Could you check a few things on this model? Use its own coordinates, in mm. A direction names the side the tool comes from. Give positions to 0.01 mm unless a question says otherwise; leave off trailing zeros. Write each loop counter-clockwise with the first axis right and the second up, starting at its lowest first coordinate (ties: lowest second). Pieces come first, ordered by that corner, then holes. Notation, with made-up numbers: M 4,70 L 17,70 A26 cw 17,99 Z; hole C 75.25,86 d11. An arc over 180 degrees is marked long. Answer as CSV lines item,"result". Start each with the question number.
from build123d import *

# Parameters (mm, degrees)
FILLET1_R           = 11
FILLET2_R           = 1
BOSS_EXTRUDE1_DEPTH = 10.425
CHAMFER1_SIZE       = 0.35


with BuildPart() as part:
    # Sketch1 → Revolve1 (revolve)
    with BuildSketch(Plane.XY, mode=Mode.PRIVATE) as revolve1_sk:
        with BuildLine():
            Line((0, 0), (8.5, 0))
            Line((8.5, 0), (8.5, 1))
            Line((8.5, 1), (5, 8))
            Line((5, 8), (4, 23))
            Line((4, 23), (3.5, 24))
            Line((3.5, 24), (2.5, 24))
            add(Edge.make_bspline(
                [(2.5, 24), (1.3, 23.5), (0, 23.5)],
                knots=[0, 0, 0, 1, 1, 1], degree=2))
            Line((0, 23.5), (0, 0))
        make_face()
    revolve(revolve1_sk.sketch.rotate(Axis((0, 23.5, 0), (0, -1, 0)), 180), axis=Axis((0, 23.5, 0), (0, -1, 0)))

    # Fillet1
    fillet1_edges = [part.edges().sort_by_distance(p)[0] for p in [
        (5, 8, 0),
    ]]
    fillet(fillet1_edges, radius=FILLET1_R)

    # Fillet2
    fillet2_edges = [part.edges().sort_by_distance(p)[0] for p in [
        (2.5, 24, 0),
        (3.5, 24, 0),
        (4, 23, 0),
        (8.5, 1, 0),
    ]]
    fillet(fillet2_edges, radius=FILLET2_R)

    # Sketch3 → Cut-Revolve1 (revolve, cut)
    with BuildSketch(Plane.XY):
        Polygon((0, 0), (3.875, 0), (3.875, 6.5), (3.05, 7.325), (3.05, 17.75), (0, 17.75), align=None)
    revolve(axis=Axis((0, 17.75, 0), (0, -1, 0)), mode=Mode.SUBTRACT)

    # Sketch4 → Boss-Extrude1 (add)
    with BuildSketch(Plane.XZ.offset(-17.75)):
        with BuildLine():
            Line((-2.655654345, 1.5), (2.655654345, 1.5))
            ThreePointArc((2.655654345, 1.5), (0, 3.05), (-2.655654345, 1.5))
        make_face()
        with BuildLine():
            ThreePointArc((-0.099986562, -3.048360656), (0, -3.05), (0.099986562, -3.048360656))
            ThreePointArc((0.099986562, -3.048360656), (0, -2.95), (-0.099986562, -3.048360656))
        make_face()
    extrude(amount=BOSS_EXTRUDE1_DEPTH)

    # Chamfer1
    # the kernel refuses this chamfer: 0.35 mm, written as the material it takes off along each edge
    with BuildSketch(Plane(origin=(-3.555743391, 7.325, 1.5), x_dir=(0, 0.9996219169112968, -0.027495876610586154), z_dir=(1, 0, 0))) as chamfer1_piece_1_section:
        Polygon((CHAMFER1_SIZE * 0.999621916911, CHAMFER1_SIZE * 0.0274958766106), (-CHAMFER1_SIZE * 0.0274958766106, CHAMFER1_SIZE * 0.999621916911), (0, 0), align=None)
    chamfer1_piece_1 = extrude(amount=7.111486782, mode=Mode.PRIVATE)
    chamfer1_piece_1 = chamfer1_piece_1 & Plane(origin=(0, 7.499624527, 0), x_dir=(1, 0, 0), z_dir=(0, 1, 0)) * Cylinder(3.05, 16, mode=Mode.PRIVATE)
    add(chamfer1_piece_1, mode=Mode.SUBTRACT)


solid = part.part
1. Thinking about a two-plate mould opening in Y: for faces 3 (the conical face through (-5.825, 5.787, -1.834)), 4 (the flat face through (4, 0, 2)), 5 (the cylindrical face through (-0.504, 3.296, 3.842)), which applies, pulls with the +Y half, pulls with the -Y half, needs draft (parallel to the pull), parting line crosses it, or undercut?
2. Imagine slicing it at A-A, the plane y = 12.5. Please give me the cut outline in (x, z), plus the area to 3 significant figures.
3. Will these pins go through, and if not, where does the flat tip stop? P1, Ø5, axis at x = 4.5, y = 4, coming from the -Z side; P2, Ø1.6, axis at x = 0, y = 15, coming from the -Z side; P3, Ø1.4, axis at x = 0, z = -0.5, coming from the -Y side.
4. On a 3-axis mill with a long thin cutter (end or side, diameter ignored), from which of +Z, -Z, +X, -X, +Y, -Y can I reach the whole of each face in a straight line? I mean faces 1 (the cylindrical face through (1.107, 0.387, -8.428)), 2 (the flat face through (0, 7.325, 2)). Say none if no direction works.
5. Imagine slicing it at B-B, the plane y = 22. Please give me the cut outline in (x, z).
6. Please list where these lines run through material, in increasing order: line 1 (Z direction, x = 0, y = 1.5) (3 decimals); line 2 (Z direction, x = -2, y = 2.5); line 3 (X direction, y = 3, z = -5).
7. Imagine slicing it at C-C, the plane y = 16.5. Please give me the cut outline in (x, z).
Solutions:
1,face 3,"pulls with the +Y half"
1,face 4,"pulls with the -Y half"
1,face 5,"needs draft"
2,outline,"C 0,0 d9.4; hole M -2.66,1.5 A3.05 ccw -0.1,-3.05 A0.1 cw 0.1,-3.05 A3.05 ccw 2.66,1.5 Z"
2,area,"46.0 mm²"
3,P1,"z = -7.42"
3,P2,"z = -4.59"
3,P3,"y = 17.75"
4,face 1,"+Y, -Y"
4,face 2,"-Y"
5,outline,"C 0,0 d8.13"
6,line 1,"-8.25 to -3.875, 3.875 to 8.25"
6,line 2,"-7.49 to -3.32, 3.32 to 7.49"
6,line 3,"-5.59 to 5.59"
7,outline,"C 0,0 d8.87; hole M -2.66,1.5 A3.05 ccw -0.1,-3.05 A0.1 cw 0.1,-3.05 A3.05 ccw 2.66,1.5 Z"
